Source: CAD feature listing. Evaluate the final solid. Frame: model axes, mm. A direction names the side the tool comes from. Round coordinates to 2 decimals unless told otherwise and drop trailing zeros. Order: outer loops, then holes, each group sorted by start corner. A loop starts at its lowest first (then second) coordinate and runs counter-clockwise, first axis right, second up. Notation, with made-up numbers: (80, 77) -> (137, 77) arc R23 ccw to (137, 116) -> close; hole circle Ø3 at (-28.75, 69.5). An arc over 180 degrees is marked (long way). Use a Markdown table: item, result. Add a question column.
```python
from build123d import *

# Parameters (mm, degrees)
F2_W     = 1000
F2_H     = 1000
F2_W_2   = 600
F2_H_2   = 800
F3_DEPTH = 18
F4_DEPTH = 300


with BuildPart() as f3:
    # F2 (on Top) → F3 (new body)
    with BuildSketch(Plane.XY):
        Rectangle(F2_W, F2_H)
        Rectangle(F2_W_2, F2_H_2, mode=Mode.SUBTRACT)
        Rectangle(F2_W_2, F2_H_2)
    extrude(amount=F3_DEPTH)

    # F2 (on Top) → F4 (join)
    with BuildSketch(Plane.XY):
        Rectangle(F2_W_2, F2_H_2)
    extrude(amount=-F4_DEPTH)


solid = f3.part
```
1) Section C-C on z = -94.5. Output: boundary loops of the cut face in (x, y), then the cut area to 3 significant figures.
2) Section B-B on y = -53. Output: boundary loops of the cut face in (x, z), then the cut area to 3 significant figures.
3) Section D-D on y = 427.5. Output: boundary loops of the cut face in (x, z).
4) Section A-A on x = -61. Output: boundary loops of the cut face in (y, z), then the cut area to 3 significant figures.
5) Reachability of faces 1 (the flat face through (-4, 400, -148)), 2 (the flat face through (300, -6, -148)), 3 (the flat face through (-4, -400, -148)) from +Z, -Z, +X, -X, +Y, -Y: full face, straight path, thin tool, end or side. Return the list, or none.
6) Line query: probe 1 along Y at (x, z) = (143, -39); probe 2 along X at (y, z) = (74, -198.5); probe 3 along Z at (x, y) = (351, 331). Output: solid intervals per line, ascending. Write a range as from..to.
7) First-contact query: pin 1 Ø1 at (x, z) = (212, -211.5) entering from +Y; pin 2 Ø5 at (y, z) = (191, -226.5) entering from -X; pin 3 Ø1 at (y, z) = (365, -17) entering from +X. Flat tips, straight axial feed; report the tip coordinate or a pass-through.
Conclusion:
| question | item | result |
|---|---|---|
| 1 | outline | (-300, -400) -> (300, -400) -> (300, 400) -> (-300, 400) -> close |
| 1 | area | 480,000 mm^2 |
| 2 | outline | (-500, 0) -> (-300, 0) -> (-300, -300) -> (300, -300) -> (300, 0) -> (500, 0) -> (500, 18) -> (-500, 18) -> close |
| 2 | area | 198,000 mm^2 |
| 3 | outline | (-500, 0) -> (500, 0) -> (500, 18) -> (-500, 18) -> close |
| 4 | outline | (-500, 0) -> (-400, 0) -> (-400, -300) -> (400, -300) -> (400, 0) -> (500, 0) -> (500, 18) -> (-500, 18) -> close |
| 4 | area | 258,000 mm^2 |
| 5 | face 1 | -Z, +X, -X, +Y |
| 5 | face 2 | -Z, +X, +Y, -Y |
| 5 | face 3 | -Z, +X, -X, -Y |
| 6 | probe 1 | y = -400..400 |
| 6 | probe 2 | x = -300..300 |
| 6 | probe 3 | z = 0..18 |
| 7 | pin 1 | stops at y = 400 |
| 7 | pin 2 | stops at x = -300 |
| 7 | pin 3 | stops at x = 300 |
